```python
from build123d import *

# Parameters (mm, degrees)
F0_R     = 1.75
F1_DEPTH = 7.5
F2_DEPTH = 4.5
F3_DEPTH = 4.5
F5_DEPTH = 8.81
F7_DEPTH = 25
F8_F1_R  = 0.5
F8_F2_R  = 0.5


with BuildPart() as f1:
    # F0 (on Top) → F1 (new body)
    with BuildSketch(Plane.XY):
        Polygon((-9.5, 0), (-5.65, 0), (5.65, 0), (9.5, 0), (9.5, 8.3), (5.65, 8.3), (5.65, 10.5504491955), (5.65, 11.4643116325), (5.65, 48), (-5.65, 48), (-5.65, 8.3), (-9.5, 8.3), align=None)
        Polygon((-5.65, 7.4641016151), (-2.65, 5.7320508076), (-2.65, 2.2679491924), (-5.65, 0.5358983849), (-8.65, 2.2679491924), (-8.65, 5.7320508076), align=None, mode=Mode.SUBTRACT)
        Polygon((2.65, 5.7320508076), (5.65, 7.4641016151), (8.65, 5.7320508076), (8.65, 2.2679491924), (5.65, 0.5358983849), (2.65, 2.2679491924), align=None, mode=Mode.SUBTRACT)
        with Locations((0, 12.25)):
            Circle(F0_R, mode=Mode.SUBTRACT)
        with BuildLine():
            ThreePointArc((-1.7499927683, 21.255030998), (0.0025155016, 22.9999981921), (1.75, 21.25))
            ThreePointArc((1.75, 21.25), (1.7499981921, 21.2474844984), (1.7499927683, 21.244969002))
            ThreePointArc((1.7499927683, 21.244969002), (-0.005030998, 19.5000072317), (-1.7499927683, 21.255030998))
        make_face(mode=Mode.SUBTRACT)
        with BuildLine():
            ThreePointArc((-1.7499927683, 33.244969002), (-0.005030998, 34.9999927683), (1.7499927683, 33.255030998))
            ThreePointArc((1.7499927683, 33.255030998), (1.7499981921, 33.2525155016), (1.75, 33.25))
            ThreePointArc((1.75, 33.25), (0.0025155016, 31.5000018079), (-1.7499927683, 33.244969002))
        make_face(mode=Mode.SUBTRACT)
        with Locations((0, 42.25)):
            Circle(F0_R, mode=Mode.SUBTRACT)
    extrude(amount=F1_DEPTH)

    # F0 (on Top) → F2 (join)
    with BuildSketch(Plane.XY):
        Polygon((-2.65, 2.2679491924), (-2.65, 5.7320508076), (-5.65, 7.4641016151), (-8.65, 5.7320508076), (-8.65, 2.2679491924), (-5.65, 0.5358983849), align=None)
        with Locations((-5.65, 4)):
            Circle(F0_R, mode=Mode.SUBTRACT)
    extrude(amount=F2_DEPTH)

    # F0 (on Top) → F3 (join)
    with BuildSketch(Plane.XY):
        Polygon((8.65, 5.7320508076), (5.65, 7.4641016151), (2.65, 5.7320508076), (2.65, 2.2679491924), (5.65, 0.5358983849), (8.65, 2.2679491924), align=None)
        with Locations((5.65, 4)):
            Circle(F0_R, mode=Mode.SUBTRACT)
    extrude(amount=F3_DEPTH)

    # F4 (on face) → F5 (cut)
    with BuildSketch(Plane.XY.offset(7.5)):
        with BuildLine():
            Line((-1.75, 21.25), (-1.75, 12.25))
            ThreePointArc((-1.75, 12.25), (0, 14), (1.75, 12.25))
            Line((1.75, 12.25), (1.75, 21.25))
            ThreePointArc((1.75, 21.25), (0, 19.5), (-1.75, 21.25))
        make_face()
    extrude(amount=-F5_DEPTH, mode=Mode.SUBTRACT)

    # F6 (on face) → F7 (cut)
    with BuildSketch(Plane.XY.offset(7.5)):
        with BuildLine():
            Line((-1.75, 42.25), (-1.75, 33.25))
            ThreePointArc((-1.75, 33.25), (0, 35), (1.75, 33.25))
            Line((1.75, 33.25), (1.75, 42.25))
            ThreePointArc((1.75, 42.25), (0, 40.5), (-1.75, 42.25))
        make_face()
    extrude(amount=-F7_DEPTH, mode=Mode.SUBTRACT)

    # F8: fillet of radius 0.5 on 20 edges, made by hand

    # F8_f1
    f8_f1_edges = [f1.edges().sort_by_distance(p)[0] for p in [
        (5.65, 8.3, 3.75),
        (-5.65, 8.3, 3.75),
    ]]
    fillet(f8_f1_edges, radius=F8_F1_R)

    # F8_f2
    f8_f2_edges = [f1.edges().sort_by_distance(p)[0] for p in [
        (-5.65, 48, 3.75),
        (5.65, 48, 3.75),
        (9.5, 8.3, 3.75),
        (-9.5, 8.3, 3.75),
        (-9.5, 0, 3.75),
        (9.5, 0, 3.75),
        (9.5, 4.15, 0),
        (9.5, 4.15, 7.5),
        (5.65, 28.4, 7.5),
        (5.65, 28.4, 0),
        (-5.65, 28.4, 0),
        (-5.65, 28.4, 7.5),
        (-9.5, 4.15, 0),
        (-9.5, 4.15, 7.5),
        (0, 48, 0),
        (0, 48, 7.5),
        (0, 0, 7.5),
        (0, 0, 0),
        (-5.7964466094, 8.4464466094, 7.5),
        (-5.7964466094, 8.4464466094, 0),
        (5.7964466094, 8.4464466094, 0),
        (5.7964466094, 8.4464466094, 7.5),
    ]]
    fillet(f8_f2_edges, radius=F8_F2_R)


solid = f1.part
```
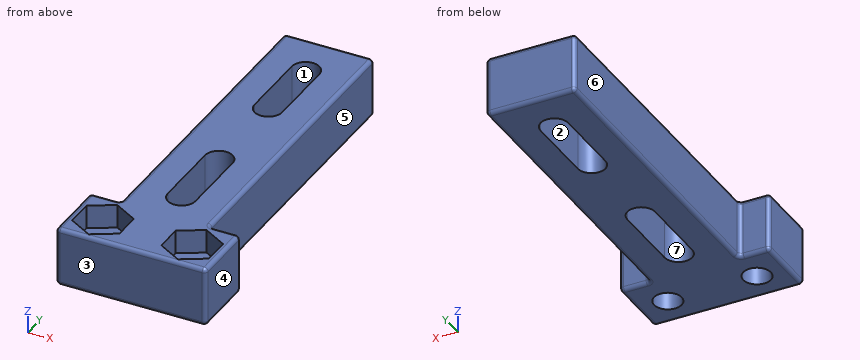
Work out the finished part from the listing and answer in its coordinate system (mm). Face numbers are marked on the shaded views. A direction names the side the tool comes from. Round coordinates to 2 decimals unless told otherwise and drop trailing zeros. Loops run counter-clockwise (first coordinate to the right, second up) from the corner with the lowest first, then second, coordinate; pieces in that order, holes last.
(1) For the marked faces 5, 6 and 7, determine the directions among +Z, -Z, +X, -X, +Y, -Y from which every point of the face is accessible in a straight line to the end or side of a thin tool.
Computed values:
face 5: +Z, -Z, +X, +Y
face 6: +Z, -Z, -X, +Y
face 7: +Z, -Z
(2) Each of these flat-tipped pins is pushed along its axis until it touches: P1, Ø0.9, axis at x = -8, z = 4, coming from the +Y side; P2, Ø3, axis at y = 28.5, z = 4.5, coming from the -X side; P3, Ø3, axis at x = 4, y = 4.5, coming from the +Z side; P4, Ø3, axis at x = -6, y = 4, coming from the +Z side. Where does it stop, or does it pass through?
Computed values:
P1: stops at y = 8.3
P2: stops at x = -5.65
P3: stops at z = 7.5
P4: stops at z = 4.5
(3) Find the intervals of material crossed by L1, parallel to X at y = 3, z = 6.5; L2, parallel to X at y = 34, z = 2.75; L3, parallel to Y at x = -1.5, z = 2.5, in increasing order.
Computed values:
L1: x = -9.5 to -8.65, -2.65 to 2.65, 8.65 to 9.5
L2: x = -5.65 to -1.75, 1.75 to 5.65
L3: y = 0 to 11.35, 22.15 to 32.35, 43.15 to 48
(4) The mould has two halves that part along X. Classify the marked faces 1, 2, 3 and 4: pulls with the +X half, pulls with the -X half, needs draft (parallel to the pull), parting line crosses it, or undercut.
Computed values:
face 1: undercut
face 2: undercut
face 3: needs draft
face 4: pulls with the +X half
(5) The part is cut by section B-B, the plane x = -0.5. Give the vertices of the cut face in (y, z), and give its area (3 significant figures).
Computed values:
outline: (0, 0.5) arc R0.5 ccw to (0.5, 0) - (10.57, 0) - (10.57, 7.5) - (0.5, 7.5) arc R0.5 ccw to (0, 7) - close; (22.93, 0) - (31.57, 0) - (31.57, 7.5) - (22.93, 7.5) - close; (43.93, 0) - (47.5, 0) arc R0.5 ccw to (48, 0.5) - (48, 7) arc R0.5 ccw to (47.5, 7.5) - (43.93, 7.5) - close
area: 174 mm2
(6) The part is cut by section A-A, the plane y = 35. Give the vertices of the cut face in (x, z).
Computed values:
outline: (-5.65, 0.5) arc R0.5 ccw to (-5.15, 0) - (-1.75, 0) - (-1.75, 7.5) - (-5.15, 7.5) arc R0.5 ccw to (-5.65, 7) - close; (1.75, 0) - (5.15, 0) arc R0.5 ccw to (5.65, 0.5) - (5.65, 7) arc R0.5 ccw to (5.15, 7.5) - (1.75, 7.5) - close
(7) The part is cut by section C-C, the plane z = 4. Give the vertices of the cut face in (x, y), and give its area (3 significant figures).
Computed values:
outline: (-9.5, 0.5) arc R0.5 ccw to (-9, 0) - (9, 0) arc R0.5 ccw to (9.5, 0.5) - (9.5, 7.8) arc R0.5 ccw to (9, 8.3) - (6.15, 8.3) arc R0.5 cw to (5.65, 8.8) - (5.65, 47.5) arc R0.5 ccw to (5.15, 48) - (-5.15, 48) arc R0.5 ccw to (-5.65, 47.5) - (-5.65, 8.8) arc R0.5 cw to (-6.15, 8.3) - (-9, 8.3) arc R0.5 ccw to (-9.5, 7.8) - close; hole circle Ø3.5 at (-5.65, 4); hole (-1.75, 12.25) arc R1.75 ccw to (1.75, 12.25) - (1.75, 21.25) arc R1.75 ccw to (-1.75, 21.25) - close; hole (-1.75, 33.25) arc R1.75 ccw to (1.75, 33.25) - (1.75, 42.25) arc R1.75 ccw to (-1.75, 42.25) - close; hole circle Ø3.5 at (5.65, 4)
area: 505 mm2
(8) The part is cut by section D-D, the plane y = 28. Give the vertices of the cut face in (x, z).
Computed values:
outline: (-5.65, 0.5) arc R0.5 ccw to (-5.15, 0) - (5.15, 0) arc R0.5 ccw to (5.65, 0.5) - (5.65, 7) arc R0.5 ccw to (5.15, 7.5) - (-5.15, 7.5) arc R0.5 ccw to (-5.65, 7) - close
